Job drawing, mm, ordinate dimensions from the low corner. One solid piece. A direction names the side the tool comes from. Coordinates: 2 decimals unless noted, no trailing zeros. Write each loop counter-clockwise with the first axis right and the second up, starting at its lowest first coordinate (ties: lowest second). Pieces come first, ordered by that corner, then holes.
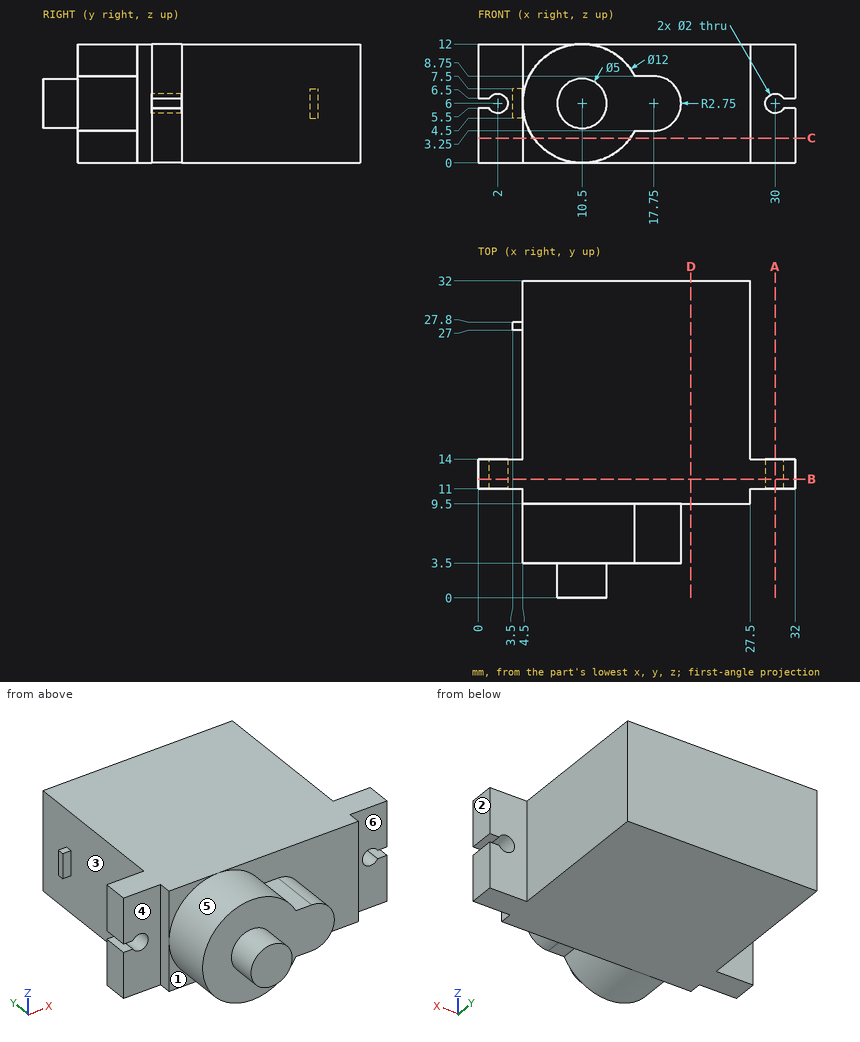
1. Saw through at B-B on y = 12. List the corners of the cut face in (x, z), plus the area to 3 significant figures.
Computed values:
outline: (0, 0) - (32, 0) - (32, 5.5) - (30.87, 5.5) arc R1 cw (long way) to (30.87, 6.5) - (32, 6.5) - (32, 12) - (0, 12) - (0, 6.5) - (1.13, 6.5) arc R1 cw (long way) to (1.13, 5.5) - (0, 5.5) - close
area: 376 mm2
2. Saw through at A-A on x = 30. List the corners of the cut face in (y, z), plus the area to 3 significant figures.
Computed values:
outline: (11, 0) - (14, 0) - (14, 5) - (11, 5) - close; (11, 7) - (14, 7) - (14, 12) - (11, 12) - close
area: 30.0 mm2
3. Flat gauge pins, fed straight in: pin 1 (1.3 mm diameter, centred on x = 3, z = 7.5, fed in from -Y); pin 2 (0.9 mm diameter, centred on x = 4, y = 27.5, fed in from -Z); pin 3 (3 mm diameter, centred on y = 21.5, z = 6.5, fed in from -X); pin 4 (1.2 mm diameter, centred on x = 31, y = 12.5, fed in from -Z). Where does each tip first touch, or does it go through?
Computed values:
pin 1: stops at y = 11
pin 2: stops at z = 4.5
pin 3: stops at x = 4.5
pin 4: stops at z = 0
4. Mould opens along Y. For the marked faces 1, 2 and 3 say: +Y half, -Y half, draft (parallel to the pull), parting line (faces both ways), or undercut.
Computed values:
face 1: -Y half
face 2: draft
face 3: undercut
5. Probe line 1 along Z through (x, y) = (2, 12); line 2 along Y through (x, z) = (20, 3.5); line 3 along X through (y, z) = (20, 5.25). List the from-to ranges inside material, lowest first.
Computed values:
line 1: z = 0 to 5, 7 to 12
line 2: y = 9.5 to 32
line 3: x = 4.5 to 27.5
6. Saw through at D-D on x = 21.5. List the corners of the cut face in (y, z).
Computed values:
outline: (9.5, 0) - (32, 0) - (32, 12) - (9.5, 12) - close
7. Saw through at C-C on z = 2.5. List the corners of the cut face in (x, y), plus the area to 3 significant figures.
Computed values:
outline: (0, 11) - (4.5, 11) - (4.5, 9.5) - (5.63, 9.5) - (5.63, 3.5) - (15.37, 3.5) - (15.37, 9.5) - (27.5, 9.5) - (27.5, 11) - (32, 11) - (32, 14) - (27.5, 14) - (27.5, 32) - (4.5, 32) - (4.5, 14) - (0, 14) - close
area: 603 mm2
8. 3-axis set-ups, long thin cutter, end or side, ignore diameter. For the marked faces 4, 5 and 6: which of +Z, -Z, +X, -X, +Y, -Y reach the whole face in a straight line?
Computed values:
face 4: +Z, -Z, -X, -Y
face 5: -Y
face 6: +Z, -Z, +X, -Y
